Geometry: final body of the model. Coordinates: model frame, mm. A direction names the side the tool comes from. Round coordinates to 2 decimals unless told otherwise and drop trailing zeros. Write each loop counter-clockwise with the first axis right and the second up, starting at its lowest first coordinate (ties: lowest second). Pieces come first, ordered by that corner, then holes. Notation, with made-up numbers: (-1, 27.25) - (48, 27.25) arc R20 ccw to (48, 59.25) - close; hole circle Ø3 at (40.5, 42). An arc over 180 degrees is marked (long way). Write each question's results on one line, items separated by ' | '.
from build123d import *

# Parameters (mm, degrees)
EXTRUDE_1_DEPTH      = 13.5
SKETCH_3_R           = 0.15
CUT_EXTRUDE_2_DEPTH  = 13.5
EXTRUDE_2_DEPTH      = 3.5
EXTRUDE_2_DEPTH_BACK = 17
EXTRUDE_3_DEPTH      = 1
EXTRUDE_3_DEPTH_BACK = 21.5
SKETCH_2_R           = 0.9
CUT_EXTRUDE_1_DEPTH  = 2.5
CUT_EXTRUDE_3_DEPTH  = 1
CUT_EXTRUDE_4_DEPTH  = 1
SKETCH_8_R           = 0.3
CUT_EXTRUDE_5_DEPTH  = 4.5
SKETCH_9_R           = 0.3
CUT_EXTRUDE_6_DEPTH  = 4.5
CUT_EXTRUDE_7_DEPTH  = 22.5


with BuildPart() as part:
    # 草图1 → 凸台-拉伸1 (new body)
    with BuildSketch(Plane(origin=(0, 0, 0), x_dir=(0, 0, -1), z_dir=(1, 0, 0))):
        Polygon((-8.5, 2.846949135), (-8.096949135, 3.25), (8.096949135, 3.25), (8.5, 2.846949135), (8.5, -2.846949135), (8.096949135, -3.25), (-8.096949135, -3.25), (-8.5, -2.846949135), align=None)
    extrude(amount=EXTRUDE_1_DEPTH)

    # 草图3 → 切除-拉伸2 (cut)
    with BuildSketch(Plane.ZY):
        with Locations((8.5, -0.253050865)):
            Circle(SKETCH_3_R)
        with Locations((-8.5, -0.253050865)):
            Circle(SKETCH_3_R)
    extrude(amount=-CUT_EXTRUDE_2_DEPTH, mode=Mode.SUBTRACT)

    # 草图4 → 凸台-拉伸2 (add, two sides)
    with BuildSketch(Plane.ZY) as extrude_2_sk:
        Polygon((8.19, -2.970178628), (8.19, 2.67), (7.91, 2.95), (-7.92, 2.95), (-8.2, 2.67), (-8.2, -2.970178628), (-7.930178628, -3.24), (7.920178628, -3.24), align=None)
    extrude(amount=EXTRUDE_2_DEPTH)
    extrude(extrude_2_sk.sketch, amount=-EXTRUDE_2_DEPTH_BACK)

    # 草图5 → 凸台-拉伸3 (add, two sides)
    with BuildSketch(Plane(origin=(17, 0, 0), x_dir=(0, 0, -1), z_dir=(1, 0, 0))) as extrude_3_sk:
        Polygon((-7.905857864, 2.94), (7.915857864, 2.94), (8.19, 2.665857864), (8.19, -2.966036493), (7.926036493, -3.23), (-7.910178628, -3.23), (-8.18, -2.960178628), (-8.18, 2.665857864), align=None)
    extrude(amount=EXTRUDE_3_DEPTH)
    extrude(extrude_3_sk.sketch, amount=-EXTRUDE_3_DEPTH_BACK)

    # 草图2 → 切除-拉伸1 (cut)
    with BuildSketch(Plane(origin=(0, 3.25, 0), x_dir=(1, 0, 0), z_dir=(0, 1, 0))):
        with Locations((2.75, 6)):
            Circle(SKETCH_2_R)
        with Locations((10.75, 6)):
            Circle(SKETCH_2_R)
        with Locations((10.75, -6)):
            Circle(SKETCH_2_R)
        with Locations((2.75, -6)):
            Circle(SKETCH_2_R)
    extrude(amount=-CUT_EXTRUDE_1_DEPTH, mode=Mode.SUBTRACT)

    # 草图6 → 切除-拉伸3 (cut)
    with BuildSketch(Plane(origin=(18, 0, 0), x_dir=(0, 0, -1), z_dir=(1, 0, 0))):
        with BuildLine():
            Line((0.3, 1.75), (0.3, 2.94))
            Line((0.3, 2.94), (-0.3, 2.94))
            Line((-0.3, 2.94), (-0.3, 1.75))
            ThreePointArc((-0.3, 1.75), (0, 1.45), (0.3, 1.75))
        make_face()
    extrude(amount=-CUT_EXTRUDE_3_DEPTH, mode=Mode.SUBTRACT)

    # 草图7 → 切除-拉伸4 (cut)
    with BuildSketch(Plane.ZY.offset(4.5)):
        with BuildLine():
            Line((-0.3, 1.75), (-0.3, 2.94))
            Line((-0.3, 2.94), (0.3, 2.94))
            Line((0.3, 2.94), (0.3, 1.75))
            ThreePointArc((0.3, 1.75), (0, 1.45), (-0.3, 1.75))
        make_face()
    extrude(amount=-CUT_EXTRUDE_4_DEPTH, mode=Mode.SUBTRACT)

    # 草图8 → 切除-拉伸5 (cut)
    with BuildSketch(Plane.ZY.offset(4.5)):
        with Locations((0, 1.75)):
            Circle(SKETCH_8_R)
    extrude(amount=-CUT_EXTRUDE_5_DEPTH, mode=Mode.SUBTRACT)

    # 草图9 → 切除-拉伸6 (cut)
    with BuildSketch(Plane(origin=(18, 0, 0), x_dir=(0, 0, -1), z_dir=(1, 0, 0))):
        with Locations((0, 1.75)):
            Circle(SKETCH_9_R)
    extrude(amount=-CUT_EXTRUDE_6_DEPTH, mode=Mode.SUBTRACT)

    # 草图10 → 切除-拉伸7 (cut)
    with BuildSketch(Plane(origin=(18, 0, 0), x_dir=(0, 0, -1), z_dir=(1, 0, 0))):
        with BuildLine():
            Line((3.497989899, -2.15), (3.497989899, -3.25))
            Line((3.497989899, -3.25), (-3.497989899, -3.25))
            Line((-3.497989899, -3.25), (-3.497989899, -2.15))
            ThreePointArc((-3.497989899, -2.15), (-3.147989899, -1.8), (-3.497989899, -1.45))
            Line((-3.497989899, -1.45), (-3.497989899, -0.85))
            Line((-3.497989899, -0.85), (-3.3, -0.652010101))
            Line((-3.3, -0.652010101), (3.3, -0.652010101))
            Line((3.3, -0.652010101), (3.497989899, -0.85))
            Line((3.497989899, -0.85), (3.497989899, -1.45))
            ThreePointArc((3.497989899, -1.45), (3.147989899, -1.8), (3.497989899, -2.15))
        make_face()
    extrude(amount=-CUT_EXTRUDE_7_DEPTH, mode=Mode.SUBTRACT)


solid = part.part
Q1. Mould query, pull axis X, two halves, no side actions, for faces 1 (the flat face through (-4.5, 0, 0)), 2 (the flat face through (-4, -3.23, -6)), 3 (the cylindrical face through (11.6, 2, -6.3)). Classes: pulls with the +X half, pulls with the -X half, needs draft (parallel to the pull), parting line crosses it, or undercut.
Answer block:
face 1: pulls with the -X half | face 2: needs draft | face 3: undercut
Q2. Access query for faces 4 (the flat face through (-2, 0, -8.2)), 5 (the cylindrical face through (3.165, 2.018, 6.798)), 6 (the flat face through (15, 0, -8.2)), 7 (the flat face through (-4, 0, 8.18)), 8 (the flat face through (-4, 2, 0.3)). Directions: +Z, -Z, +X, -X, +Y, -Y. A direction counts if a zero-diameter tool reaches every point of the face in a straight line with its end or side. Return the directions, or none.
Answer block:
face 4: -Z, -X, +Y, -Y | face 5: +Y | face 6: -Z, +X, +Y, -Y | face 7: +Z, -X, +Y, -Y | face 8: -X, +Y
Q3. Section query A-A, the plane x = 16.75. Return loops of the section in (y, z), plus the area to 3 significant figures.
Answer block:
outline: (-3.24, -7.93) - (-2.97, -8.2) - (2.67, -8.2) - (2.95, -7.92) - (2.95, 7.91) - (2.67, 8.19) - (-2.97, 8.19) - (-3.24, 7.92) - (-3.24, 3.5) - (-2.15, 3.5) arc R0.35 ccw to (-1.45, 3.5) - (-0.85, 3.5) - (-0.65, 3.3) - (-0.65, -3.3) - (-0.85, -3.5) - (-1.45, -3.5) arc R0.35 ccw to (-2.15, -3.5) - (-3.24, -3.5) - close; hole circle Ø0.6 at (1.75, 0) | area: 83.3 mm2
Q4. Section query D-D, the plane x = 9. Return loops of the section in (y, z), plus the area to 3 significant figures.
Answer block:
outline: (-3.25, -8.1) - (-2.85, -8.5) - (-0.4, -8.5) arc R0.15 cw to (-0.1, -8.5) - (2.85, -8.5) - (3.25, -8.1) - (3.25, 8.1) - (2.85, 8.5) - (-0.1, 8.5) arc R0.15 cw to (-0.4, 8.5) - (-2.85, 8.5) - (-3.25, 8.1) - (-3.25, 3.5) - (-2.15, 3.5) arc R0.35 ccw to (-1.45, 3.5) - (-0.85, 3.5) - (-0.65, 3.3) - (-0.65, -3.3) - (-0.85, -3.5) - (-1.45, -3.5) arc R0.35 ccw to (-2.15, -3.5) - (-3.25, -3.5) - close | area: 92.4 mm2
Q5. Pin query (flat end, axial travel): pin 1 (2 mm diameter, centred on x = 10, z = 0, fed in from -Y); pin 2 (0.8 mm diameter, centred on x = 17.5, y = 2.5, fed in from +Z); pin 3 (0.8 mm diameter, centred on x = -4, y = 2, fed in from -Z). Return the tip coordinate at first contact, or that it passes through.
Answer block:
pin 1: y = -0.65 | pin 2: z = 8.18 | pin 3: z = -8.19
Q6. Ray query, line 1 along X through (y, z) = (2.75, 6); line 2 along Z through (x, y) = (2.75, 1.55); line 3 along Z through (x, y) = (9.5, -1.75). Return the intervals inside material, ascending.
Answer block:
line 1: -4.5 to 1.85, 3.65 to 9.85, 11.65 to 18 | line 2: -8.5 to -6.9, -5.1 to 5.1, 6.9 to 8.5 | line 3: -8.5 to -3.15, 3.15 to 8.5
